CAD build for the part. Positions are in the model's coordinates, mm. Face numbers are marked on the shaded views. A direction names the side the tool comes from. Coordinates: 2 decimals unless noted, no trailing zeros. Write each loop counter-clockwise with the first axis right and the second up, starting at its lowest first coordinate (ties: lowest second). Pieces come first, ordered by that corner, then holes. Notation, with made-up numbers: (58, 69.25) - (73, 69.25) arc R27 ccw to (73, 85.25) - close; hole circle Ø9 at (19, 3.5). An arc over 180 degrees is marked (long way). One line per question, with ' | ' between items. Start each with the question number.
1. Which spindle directions (+Z, -Z, +X, -X, +Y, -Y) get a long thin tool onto all of the face, cutting with end or side? Do the marked faces 5, 6, 7 and 8. Say none if no direction does.
2. Probe line 1 (X direction, y = -18, z = 29); line 2 (Y direction, x = 10, z = 103.9); line 3 (X direction, y = 23, z = 87). List the from-to ranges inside material, lowest first.
3. Flat gauge pins, fed straight in: P1, Ø4, axis at x = 10, z = 87, coming from the +Y side; P2, Ø4.5, axis at y = 43, z = 104, coming from the +X side; P3, Ø1, axis at x = -23.5, y = 13.5, coming from the +Z side. Where does each tip first touch, or does it go through?
4. Band-saw the part on B-B, the plane z = 87. Write the cut outline in (x, y).
5. Band-saw the part on D-D, the plane y = 36.5. Write the cut outline in (x, z).
6. Band-saw the part on A-A, the plane x = 30. Write the cut outline in (y, z).
7. Band-saw the part on C-C, the plane z = 25.5. Write the cut outline in (x, y).
8. Two-plate mould, pull along Z, no slides. Class the marked faces 1, 2, 3 and 4: +Z half, -Z half, draft (parallel to the pull), parting line (faces both ways), or undercut.
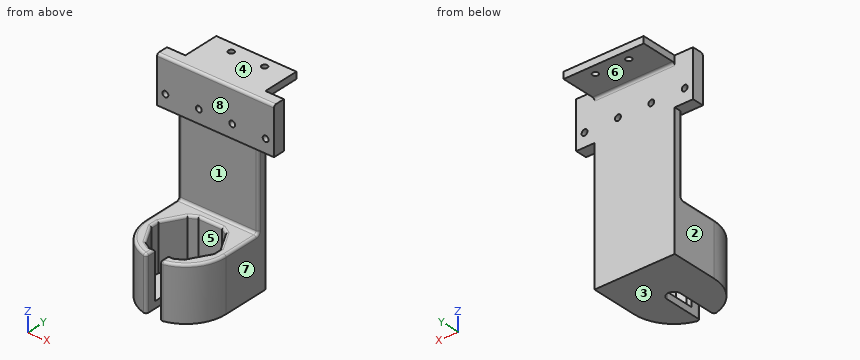
from build123d import *

# Parameters (mm, degrees)
SKETCH1_R                = 24
BOSS_EXTRUDE2_DEPTH      = 32
CUT_EXTRUDE1_DEPTH       = 28
CUT_EXTRUDE2_REACH       = 48.648
SKETCH3_W                = 8
SKETCH3_H                = 8
BOSS_EXTRUDE3_DEPTH      = 32
SKETCH6_W                = 48
SKETCH6_H                = 5
BOSS_EXTRUDE4_DEPTH      = 75
SKETCH7_W                = 48
SKETCH7_H                = 4
BOSS_EXTRUDE5_DEPTH      = 22
CUT_EXTRUDE3_REACH       = 118.983
SKETCH8_R                = 1.75
BOSS_EXTRUDE7_DEPTH      = 2
BOSS_EXTRUDE7_DEPTH_BACK = 5
SKETCH11_W               = 70
SKETCH11_H               = 28
CUT_EXTRUDE5_REACH       = 126.008
SKETCH12_R               = 1.75
CUT_EXTRUDE6_DEPTH       = 97.695398029
FILLET2_R                = 1.5
FILLET3_R                = 4


with BuildPart() as part:
    # Sketch1 → Boss-Extrude2 (new body)
    with BuildSketch(Plane(origin=(0, 0, 0), x_dir=(0, 1, 0), z_dir=(0, 0, 1))):
        with Locations(Location((0, 0, 0), (0, 0, 270))):
            Circle(SKETCH1_R)
    extrude(amount=BOSS_EXTRUDE2_DEPTH)

    # Sketch2 → Cut-Extrude1 (cut)
    with BuildSketch(Plane.XY.offset(32)):
        Polygon((7.09995, 17.23849547), (-7.09995, 17.23849547), (-11.379, 14.767984801), (-18.47895, 2.470510669), (-18.47895, -2.470510669), (-11.379, -14.767984801), (-7.09995, -17.23849547), (7.09995, -17.23849547), (11.379, -14.767984801), (18.47895, -2.470510669), (18.47895, 2.470510669), (11.379, 14.767984801), align=None)
    extrude(amount=-CUT_EXTRUDE1_DEPTH, mode=Mode.SUBTRACT)

    # Sketch3 → Cut-Extrude2 (cut, up to next)
    with BuildSketch(Plane(origin=(0, 0, 0), x_dir=(1, 0, 0), z_dir=(0, 0, -1)), mode=Mode.PRIVATE) as cut_extrude2_sk1:
        Rectangle(SKETCH3_W, SKETCH3_H)
    cut_extrude2_tool1 = extrude(cut_extrude2_sk1.sketch, amount=-CUT_EXTRUDE2_REACH, mode=Mode.PRIVATE) & part.part
    add(cut_extrude2_tool1.solids().sort_by_distance((0, 0, 0))[0], mode=Mode.SUBTRACT)

    # Sketch4 → Boss-Extrude3 (add)
    with BuildSketch(Plane.XY.offset(32)):
        with BuildLine():
            Line((-24, 0), (-24, 28))
            Line((-24, 28), (24, 28))
            Line((24, 28), (24, 0))
            Line((24, 0), (22, 0))
            ThreePointArc((22, 0), (0, 22), (-22, 0))
            Line((-22, 0), (-24, 0))
        make_face()
    extrude(amount=-BOSS_EXTRUDE3_DEPTH)

    # Sketch6 → Boss-Extrude4 (add)
    with BuildSketch(Plane.XY.offset(32)):
        with Locations((0, 25.5)):
            Rectangle(SKETCH6_W, SKETCH6_H)
    extrude(amount=BOSS_EXTRUDE4_DEPTH)

    # Sketch7 → Boss-Extrude5 (add)
    with BuildSketch(Plane(origin=(0, 28, 0), x_dir=(-1, 0, 0), z_dir=(0, 1, 0))):
        with Locations((0, 105)):
            Rectangle(SKETCH7_W, SKETCH7_H)
    extrude(amount=BOSS_EXTRUDE5_DEPTH)

    # Sketch8 → Cut-Extrude3 (cut, up to next)
    with BuildSketch(Plane(origin=(0, 0, 103), x_dir=(1, 0, 0), z_dir=(0, 0, -1)), mode=Mode.PRIVATE) as cut_extrude3_sk1:
        with Locations(Location((-10, -44, 0), (0, 0, 180))):
            Circle(SKETCH8_R)
    cut_extrude3_tool1 = extrude(cut_extrude3_sk1.sketch, amount=-CUT_EXTRUDE3_REACH, mode=Mode.PRIVATE) & part.part
    # Sketch8 → Cut-Extrude3 (cut, up to next)
    with BuildSketch(Plane(origin=(0, 0, 103), x_dir=(1, 0, 0), z_dir=(0, 0, -1)), mode=Mode.PRIVATE) as cut_extrude3_sk2:
        with Locations((10, -44)):
            Circle(SKETCH8_R)
    cut_extrude3_tool2 = extrude(cut_extrude3_sk2.sketch, amount=-CUT_EXTRUDE3_REACH, mode=Mode.PRIVATE) & part.part
    add(cut_extrude3_tool1.solids().sort_by_distance((-10, 44, 103))[0], mode=Mode.SUBTRACT)
    add(cut_extrude3_tool2.solids().sort_by_distance((10, 44, 103))[0], mode=Mode.SUBTRACT)

    # Sketch11 → Boss-Extrude7 (add, two sides: drawn at the far end of the back side and taken through both)
    with BuildSketch(Plane.XZ.offset(-23).offset(-BOSS_EXTRUDE7_DEPTH_BACK)):
        with Locations((0, 93)):
            Rectangle(SKETCH11_W, SKETCH11_H)
    extrude(amount=BOSS_EXTRUDE7_DEPTH + BOSS_EXTRUDE7_DEPTH_BACK)

    # Sketch12 → Cut-Extrude5 (cut, up to next)
    with BuildSketch(Plane(origin=(0, 28, 0), x_dir=(-1, 0, 0), z_dir=(0, 1, 0)), mode=Mode.PRIVATE) as cut_extrude5_sk1:
        with Locations(Location((-10, 87, 0), (0, 0, 90))):
            Circle(SKETCH12_R)
    cut_extrude5_tool1 = extrude(cut_extrude5_sk1.sketch, amount=-CUT_EXTRUDE5_REACH, mode=Mode.PRIVATE) & part.part
    # Sketch12 → Cut-Extrude5 (cut, up to next)
    with BuildSketch(Plane(origin=(0, 28, 0), x_dir=(-1, 0, 0), z_dir=(0, 1, 0)), mode=Mode.PRIVATE) as cut_extrude5_sk2:
        with Locations(Location((-30, 87, 0), (0, 0, 90))):
            Circle(SKETCH12_R)
    cut_extrude5_tool2 = extrude(cut_extrude5_sk2.sketch, amount=-CUT_EXTRUDE5_REACH, mode=Mode.PRIVATE) & part.part
    # Sketch12 → Cut-Extrude5 (cut, up to next)
    with BuildSketch(Plane(origin=(0, 28, 0), x_dir=(-1, 0, 0), z_dir=(0, 1, 0)), mode=Mode.PRIVATE) as cut_extrude5_sk3:
        with Locations(Location((10, 87, 0), (0, 0, 270))):
            Circle(SKETCH12_R)
    cut_extrude5_tool3 = extrude(cut_extrude5_sk3.sketch, amount=-CUT_EXTRUDE5_REACH, mode=Mode.PRIVATE) & part.part
    # Sketch12 → Cut-Extrude5 (cut, up to next)
    with BuildSketch(Plane(origin=(0, 28, 0), x_dir=(-1, 0, 0), z_dir=(0, 1, 0)), mode=Mode.PRIVATE) as cut_extrude5_sk4:
        with Locations(Location((30, 87, 0), (0, 0, 270))):
            Circle(SKETCH12_R)
    cut_extrude5_tool4 = extrude(cut_extrude5_sk4.sketch, amount=-CUT_EXTRUDE5_REACH, mode=Mode.PRIVATE) & part.part
    add(cut_extrude5_tool1.solids().sort_by_distance((10, 28, 87))[0], mode=Mode.SUBTRACT)
    add(cut_extrude5_tool2.solids().sort_by_distance((30, 28, 87))[0], mode=Mode.SUBTRACT)
    add(cut_extrude5_tool3.solids().sort_by_distance((-10, 28, 87))[0], mode=Mode.SUBTRACT)
    add(cut_extrude5_tool4.solids().sort_by_distance((-30, 28, 87))[0], mode=Mode.SUBTRACT)

    # Sketch13 → Cut-Extrude6 (cut, through all)
    with BuildSketch(Plane.XY.offset(32)):
        with BuildLine():
            Line((-4, -4), (-4, -23.664319132))
            ThreePointArc((-4, -23.664319132), (0, -24), (4, -23.664319132))
            Line((4, -23.664319132), (4, -4))
            Line((4, -4), (-4, -4))
        make_face()
    extrude(amount=-CUT_EXTRUDE6_DEPTH, mode=Mode.SUBTRACT)

    # Fillet2
    fillet2_edges = [part.edges().sort_by_distance(p)[0] for p in [
        (24, 23, 55.5),
        (-24, 23, 55.5),
        (0, 21, 107),
        (-9.239475, 16.003240135, 32),
        (-14.928975, 8.619247735, 32),
        (5.549975, -17.23849547, 32),
        (-18.47895, 0, 32),
        (18.33030278, -15.491933385, 32),
        (-14.928975, -8.619247735, 32),
        (-4, -20.451407301, 32),
        (4, -20.451407301, 32),
        (-9.239475, -16.003240135, 32),
        (4, -23.664319132, 16),
        (-4, -23.664319132, 16),
        (-5.549975, -17.23849547, 32),
        (9.239475, -16.003240135, 32),
        (14.928975, -8.619247735, 32),
        (18.47895, 0, 32),
        (14.928975, 8.619247735, 32),
        (9.239475, 16.003240135, 32),
        (0, 17.23849547, 32),
        (-18.33030278, -15.491933385, 32),
        (24, 11.5, 32),
        (-24, 11.5, 32),
        (0, 23, 32),
        (0, 28, 103),
    ]]
    fillet(fillet2_edges, radius=FILLET2_R)

    # Fillet3
    fillet3_edges = [part.edges().sort_by_distance(p)[0] for p in [
        (-4, 4, 2),
        (4, 4, 2),
    ]]
    fillet(fillet3_edges, radius=FILLET3_R - 0.0001)  # a hair under: the kernel refuses the full size


solid = part.part
Filled in:
1) face 5: +Z | face 6: -Z, +X, -X, +Y | face 7: -Z, +X, +Y, -Y | face 8: +Z, +X, -X, -Y
2) line 1: x = -15.87 to -4, 4 to 15.87 | line 2: y = 21 to 42.25, 45.75 to 50 | line 3: x = -35 to -31.75, -28.25 to -11.75, -8.25 to 8.25, 11.75 to 28.25, 31.75 to 35
3) P1: stops at y = 28 | P2: stops at x = 24 | P3: stops at z = 31.91
4) outline: (-35, 21) - (-31.75, 21) - (-31.75, 28) - (-35, 28) - close; (-28.25, 21) - (-11.75, 21) - (-11.75, 28) - (-28.25, 28) - close; (-8.25, 21) - (8.25, 21) - (8.25, 28) - (-8.25, 28) - close; (11.75, 21) - (28.25, 21) - (28.25, 28) - (11.75, 28) - close; (31.75, 21) - (35, 21) - (35, 28) - (31.75, 28) - close
5) outline: (-24, 103) - (24, 103) - (24, 107) - (-24, 107) - close
6) outline: (21, 79) - (28, 79) - (28, 85.25) - (21, 85.25) - close; (21, 88.75) - (28, 88.75) - (28, 107) - (22.5, 107) arc R1.5 ccw to (21, 105.5) - close
7) outline: (-24, 0) arc R24 ccw to (-5.87, -23.27) arc R1.5 ccw to (-4, -21.82) - (-4, -17.24) - (-7.1, -17.24) - (-11.38, -14.77) - (-18.48, -2.47) - (-18.48, 2.47) - (-11.38, 14.77) - (-7.1, 17.24) - (7.1, 17.24) - (11.38, 14.77) - (18.48, 2.47) - (18.48, -2.47) - (11.38, -14.77) - (7.1, -17.24) - (4, -17.24) - (4, -21.82) arc R1.5 ccw to (5.87, -23.27) arc R24 ccw to (24, 0) - (24, 28) - (-24, 28) - close
8) face 1: undercut | face 2: draft | face 3: -Z half | face 4: +Z half
